Verification items for this drawing (mm, ordinates from the low corner). Round coordinates to 2 decimals unless told otherwise and drop trailing zeros. Order: outer loops, then holes, each group sorted by start corner. A loop starts at its lowest first (then second) coordinate and runs counter-clockwise, first axis right, second up. Notation, with made-up numbers: (73, -29) - (97, -29) arc R25 cw to (97, 1) - close; hole circle Ø1 at (14, 72.25). An arc over 180 degrees is marked (long way). Use a Markdown table: item, result. Add a question column.
(1) Section check C-C on y = 1.85. Record the boundary of the cut face in (x, z) (3 decimals).
(2) Section check B-B on z = 12.7. Record the boundary of the cut face in (x, y) (3 decimals), then the cut area to 3 significant figures.
(3) Thickness scan on line 1 along X through (y, z) = (1.55, 12.5); line 2 along Z through (x, y) = (38.1, 2.15) (3 decimals); line 3 along X through (y, z) = (0.35, 11). Record the ranges inside material, lowest first. Write a range as [from, to].
(4) Section check A-A on x = 139.7. Record the boundary of the cut face in (y, z) (3 decimals), then the cut area to 3 significant figures.
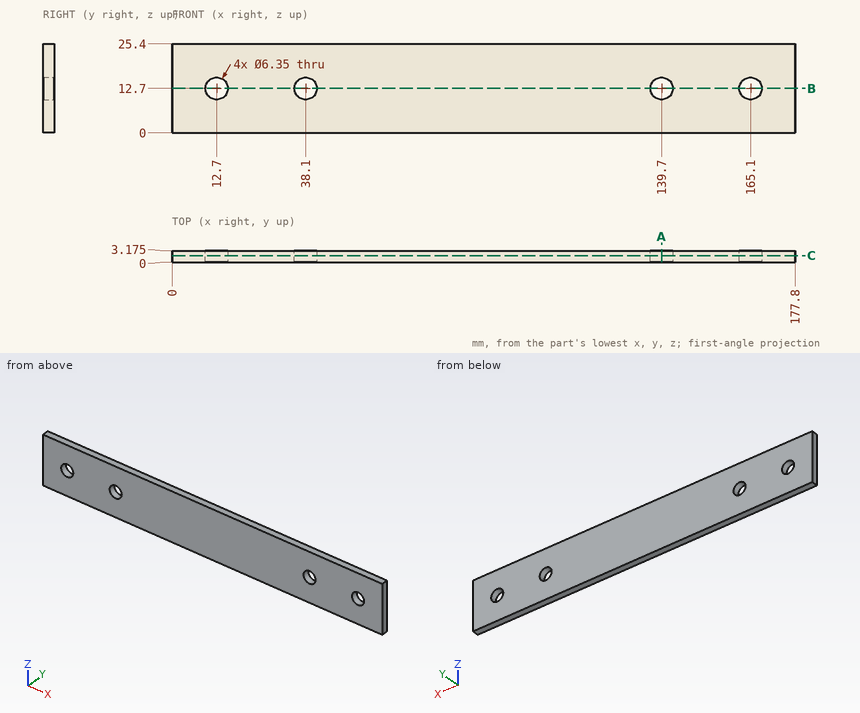
Check sheet entries:
| question | item | result |
|---|---|---|
| 1 | outline | (0, 0) - (177.8, 0) - (177.8, 25.4) - (0, 25.4) - close; hole circle Ø6.35 at (12.7, 12.7); hole circle Ø6.35 at (38.1, 12.7); hole circle Ø6.35 at (139.7, 12.7); hole circle Ø6.35 at (165.1, 12.7) |
| 2 | outline | (0, 0) - (9.525, 0) - (9.525, 3.175) - (0, 3.175) - close; (15.875, 0) - (34.925, 0) - (34.925, 3.175) - (15.875, 3.175) - close; (41.275, 0) - (136.525, 0) - (136.525, 3.175) - (41.275, 3.175) - close; (142.875, 0) - (161.925, 0) - (161.925, 3.175) - (142.875, 3.175) - close; (168.275, 0) - (177.8, 0) - (177.8, 3.175) - (168.275, 3.175) - close |
| 2 | area | 484 mm2 |
| 3 | line 1 | x = [0, 9.53], [15.87, 34.93], [41.27, 136.53], [142.87, 161.93], [168.27, 177.8] |
| 3 | line 2 | z = [0, 9.525], [15.875, 25.4] |
| 3 | line 3 | x = [0, 10.02], [15.38, 35.42], [40.78, 137.02], [142.38, 162.42], [167.78, 177.8] |
| 4 | outline | (0, 0) - (3.175, 0) - (3.175, 9.525) - (0, 9.525) - close; (0, 15.875) - (3.175, 15.875) - (3.175, 25.4) - (0, 25.4) - close |
| 4 | area | 60.5 mm2 |
